from build123d import *

# Parameters (mm, degrees)
SKETCH1_R           = 3.175
BOSS_EXTRUDE1_DEPTH = 6.35
CHAMFER1_SIZE       = 3.175


with BuildPart() as part:
    # Sketch1 → Boss-Extrude1 (new body)
    with BuildSketch(Plane.XZ.offset(109.25)):
        with BuildLine():
            ThreePointArc((-94.300070948, -79.127154752), (-66.095055559, -119.40809126), (-45.31324895, -163.974819355))
            Line((-45.31324895, -163.974819355), (-35.802288852, -190.105967461))
            ThreePointArc((-35.802288852, -190.105967461), (0, -215.175), (35.802288852, -190.105967461))
            Line((35.802288852, -190.105967461), (45.31324895, -163.974819355))
            ThreePointArc((45.31324895, -163.974819355), (66.095055559, -119.40809126), (94.300070948, -79.127154752))
            ThreePointArc((94.300070948, -79.127154752), (0, 123.1), (-94.300070948, -79.127154752))
        make_face()
        with Locations(Location((-47.329330924, -142.15, 0), (0, 0, 270))):
            Circle(SKETCH1_R, mode=Mode.SUBTRACT)
        with Locations(Location((-82.554716704, -82.554716704, 0), (0, 0, 270))):
            Circle(SKETCH1_R, mode=Mode.SUBTRACT)
        with Locations(Location((0, -208.825, 0), (0, 0, 270))):
            Circle(SKETCH1_R, mode=Mode.SUBTRACT)
        with Locations(Location((47.329330924, -142.15, 0), (0, 0, 270))):
            Circle(SKETCH1_R, mode=Mode.SUBTRACT)
        with Locations(Location((82.554716704, -82.554716704, 0), (0, 0, 270))):
            Circle(SKETCH1_R, mode=Mode.SUBTRACT)
        with Locations(Location((-116.75, 0, 0), (0, 0, 270))):
            Circle(SKETCH1_R, mode=Mode.SUBTRACT)
        with Locations(Location((-82.554716704, 82.554716704, 0), (0, 0, 270))):
            Circle(SKETCH1_R, mode=Mode.SUBTRACT)
        with Locations(Location((116.75, 0, 0), (0, 0, 270))):
            Circle(SKETCH1_R, mode=Mode.SUBTRACT)
        with Locations(Location((0, 116.75, 0), (0, 0, 270))):
            Circle(SKETCH1_R, mode=Mode.SUBTRACT)
        with Locations(Location((82.554716704, 82.554716704, 0), (0, 0, 270))):
            Circle(SKETCH1_R, mode=Mode.SUBTRACT)
    extrude(amount=BOSS_EXTRUDE1_DEPTH)

    # Chamfer1
    chamfer1_edges = [part.edges().sort_by_distance(p)[0] for p in [
        (0, -115.6, -205.65),
        (82.554716704, -115.6, 85.729716704),
        (-82.554716704, -115.6, -79.379716704),
        (-82.554716704, -115.6, 85.729716704),
        (82.554716704, -115.6, -79.379716704),
    ]]
    chamfer(chamfer1_edges, length=CHAMFER1_SIZE - 0.0001)  # a hair under: the kernel refuses the full size


solid = part.part
Source: CAD feature listing. Evaluate the final solid. Frame: model axes, mm. Coordinates: 2 decimals unless noted, no trailing zeros. Loops run counter-clockwise (first coordinate to the right, second up) from the corner with the lowest first, then second, coordinate; pieces in that order, holes last. Notation, with made-up numbers: (-35.5, 25.5) - (11.5, 25.5) arc R23 ccw to (11.5, 61.5) - close; hole circle Ø2 at (-33, 27). An arc over 180 degrees is marked (long way). One line per item, written item: value. Start each with the question number.
1. Section C-C (z = 69). Return the cut outline in (x, y).
2. Contact query for flat-ended pins moving along their axis: P1, Ø1.5, axis at x = 80, y = -110, coming from the +Z side; P2, Ø2, axis at y = -110, z = 42.5, coming from the +X side; P3, Ø1, axis at x = -9, y = -113, coming from the +Z side. Output: stop coordinate, or through.
3. Section A-A (y = -111.25). State how many separate pieces and enclosed holes the cut face has, and give its area (3 significant figures).
4. Ray query, L1, parallel to X at y = -112.25, z = 0 (3 decimals); L2, parallel to X at y = -115, z = 14; L3, parallel to X at y = -113.25, z = 28. Return the intervals inside material, ascending.
5. Section B-B (x = 100). Return the cut outline in (y, z).
6. Mould query, pull axis X, two halves, no side actions, for faces 1 (the flat face through (40.5, -112.4, -177.2)), 2 (the flat face through (-40.624, -112.381, -176.857)), 3 (the conical face through (85.9, -112.624, -82.116)). Classes: pulls with the +X half, pulls with the -X half, needs draft (parallel to the pull), parting line crosses it, or undercut.
Verdict:
1. outline: (-101.94, -115.6) - (101.94, -115.6) - (101.94, -109.25) - (-101.94, -109.25) - close
2. P1: stops at z = 94.2
2. P2: stops at x = 115.89
2. P3: stops at z = 122.81
3. separate pieces: 1
3. enclosed holes: 10
3. area: 56,200 mm2
4. L1: x = -123.1 to -119.925, -113.575 to 113.575, 119.925 to 123.1
4. L2: x = -122.3 to 122.3
4. L3: x = -119.87 to 119.87
5. outline: (-115.6, -71.79) - (-109.25, -71.79) - (-109.25, 71.79) - (-115.6, 71.79) - close
6. face 1: pulls with the +X half
6. face 2: pulls with the -X half
6. face 3: undercut
